```python
from build123d import *

# Parameters (mm, degrees)
SKETCH002_W     = 18
SKETCH002_H     = 115
SKETCH002_R     = 1.35
PAD001_DEPTH    = 4.6
POCKET001_DEPTH = 2.6
FILLET001_R     = 7


with BuildPart() as part:
    # Sketch002 → Pad001 (new body)
    with BuildSketch(Plane.XY):
        Rectangle(SKETCH002_W, SKETCH002_H)
        with Locations((0, 51.5)):
            Circle(SKETCH002_R, mode=Mode.SUBTRACT)
        with Locations((0, -51.5)):
            Circle(SKETCH002_R, mode=Mode.SUBTRACT)
    extrude(amount=PAD001_DEPTH)

    # Sketch003 (on Face7 of Pad001) → Pocket001 (cut)
    with BuildSketch(Plane(origin=(0, 0, 0), x_dir=(1, 0, 0), z_dir=(0, 0, -1))):
        Polygon((2.684679, 49.95), (2.684679, 53.05), (0, 54.6), (-2.684679, 53.05), (-2.684679, 49.95), (0, 48.4), align=None)
        Polygon((2.684679, -53.05), (2.684679, -49.95), (0, -48.4), (-2.684679, -49.95), (-2.684679, -53.05), (0, -54.6), align=None)
    extrude(amount=-POCKET001_DEPTH, mode=Mode.SUBTRACT)

    # Fillet001
    fillet001_edges = [part.edges().sort_by_distance(p)[0] for p in [
        (-9, 57.5, 2.3),
        (9, 57.5, 2.3),
        (9, -57.5, 2.3),
        (-9, -57.5, 2.3),
    ]]
    fillet(fillet001_edges, radius=FILLET001_R)


solid = part.part
```
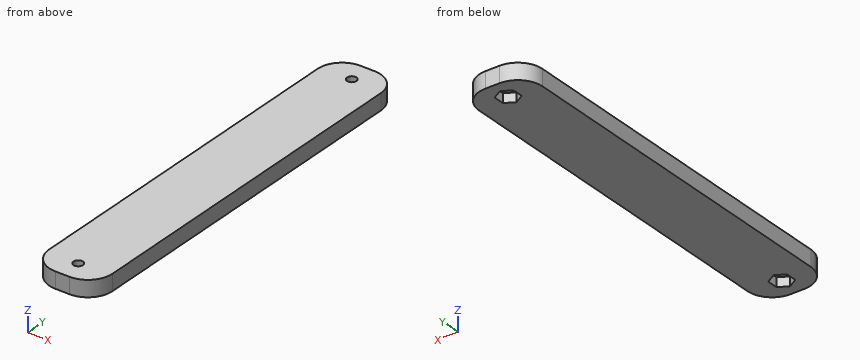
For this review, take the finished solid that the model builds, in its own axes (mm). Give positions to 0.01 mm unless a question says otherwise; leave off trailing zeros. Order: outer loops, then holes, each group sorted by start corner. A loop starts at its lowest first (then second) coordinate and runs counter-clockwise, first axis right, second up.
1) Wall thickness on line 1 (Y direction, x = 0, z = 3.75); line 2 (Y direction, x = 0, z = 2.15); line 3 (Y direction, x = 2.25, z = 3.15): over which ranges is each line inside the solid? List them lowest first.
2) Insertion check: pin 1 (6 mm diameter, centred on x = -0.5, y = -50.5, fed in from -Z); pin 2 (3 mm diameter, centred on x = 0, y = 51.5, fed in from -Z); pin 3 (1 mm diameter, centred on x = -5, z = 4, fed in from -Y); pin 4 (0.8 mm diameter, centred on y = 51.5, z = 1.5, fed in from +X). Each pin has a flat end and moves straight along its axis. Give the tip position at first contact, or say it passes through.
3) Take a section at C-C (x = 5.5). Give the boundary of the cut face in (y, z), then the cut area to 3 significant figures.
4) Take a section at A-A (z = 3.4). Give the boundary of the cut face in (x, y).
5) Take a section at B-B (y = -51.5). Give the boundary of the cut face in (x, z), then the cut area to 3 significant figures.
Derived:
1. line 1: y = -57.5 to -52.85, -50.15 to 50.15, 52.85 to 57.5
1. line 2: y = -57.5 to -54.6, -48.4 to 48.4, 54.6 to 57.5
1. line 3: y = -57.5 to 57.5
2. pin 1: stops at z = 0
2. pin 2: stops at z = 2.6
2. pin 3: stops at y = -57.04
2. pin 4: stops at x = 8.97
3. outline: (-56.56, 0) - (56.56, 0) - (56.56, 4.6) - (-56.56, 4.6) - close
3. area: 520 mm2
4. outline: (-9, -50.5) arc R7 ccw to (-2, -57.5) - (2, -57.5) arc R7 ccw to (9, -50.5) - (9, 50.5) arc R7 ccw to (2, 57.5) - (-2, 57.5) arc R7 ccw to (-9, 50.5) - close; hole circle Ø2.7 at (0, -51.5); hole circle Ø2.7 at (0, 51.5)
5. outline: (-8.93, 0) - (-2.68, 0) - (-2.68, 2.6) - (-1.35, 2.6) - (-1.35, 4.6) - (-8.93, 4.6) - close; (1.35, 2.6) - (2.68, 2.6) - (2.68, 0) - (8.93, 0) - (8.93, 4.6) - (1.35, 4.6) - close
5. area: 62.8 mm2
